```python
from build123d import *

# Parameters (mm, degrees)
SKETCH1_R           = 1.5
SKETCH1_R_2         = 10.079418918
BOSS_EXTRUDE1_DEPTH = 5
SKETCH2_W           = 5
SKETCH2_H           = 27
BOSS_EXTRUDE2_DEPTH = 39
SKETCH3_W           = 10
SKETCH3_H           = 27
SKETCH3_R           = 2
BOSS_EXTRUDE3_DEPTH = 3


with BuildPart() as part:
    # Sketch1 → Boss-Extrude1 (new body)
    with BuildSketch(Plane(origin=(0, 0, 0), x_dir=(1, 0, 0), z_dir=(0, 1, 0))):
        with BuildLine():
            Line((41.602990033, 18.779069767), (4.519397898, 18.779069767))
            ThreePointArc((4.519397898, 18.779069767), (-8.897009967, 24.779069767), (-22.313417832, 18.779069767))
            Line((-22.313417832, 18.779069767), (-31.397009967, 18.779069767))
            Line((-31.397009967, 18.779069767), (-31.397009967, -8.220930233))
            Line((-31.397009967, -8.220930233), (41.602990033, -8.220930233))
            Line((41.602990033, -8.220930233), (41.602990033, 18.779069767))
        make_face()
        with BuildLine():
            ThreePointArc((-23.542908001, -3.720930233), (-23.535781037, -3.712942946), (-23.528673093, -3.704938729))
            ThreePointArc((-23.528673093, -3.704938729), (-23.522939474, -3.712936049), (-23.517201484, -3.720930233))
            Line((-23.517201484, -3.720930233), (-23.542908001, -3.720930233))
        make_face(mode=Mode.SUBTRACT)
        with Locations(Location((-26.897009967, -0.720930233, 0), (0, 0, 270))):
            Circle(SKETCH1_R, mode=Mode.SUBTRACT)
        with Locations(Location((37.102990033, -3.720930233, 0), (0, 0, 270))):
            Circle(SKETCH1_R, mode=Mode.SUBTRACT)
        with Locations(Location((-8.897009967, 6.779069767, 0), (0, 0, 270))):
            Circle(SKETCH1_R_2, mode=Mode.SUBTRACT)
        with Locations(Location((9.102990033, 14.279069767, 0), (0, 0, 270))):
            Circle(SKETCH1_R, mode=Mode.SUBTRACT)
    extrude(amount=BOSS_EXTRUDE1_DEPTH)

    # Sketch2 → Boss-Extrude2 (add)
    with BuildSketch(Plane(origin=(0, 5, 0), x_dir=(1, 0, 0), z_dir=(0, 1, 0))):
        with Locations((-33.897009967, 5.279069767)):
            Rectangle(SKETCH2_W, SKETCH2_H)
        with Locations((44.102990033, 5.279069767)):
            Rectangle(SKETCH2_W, SKETCH2_H)
    extrude(amount=-BOSS_EXTRUDE2_DEPTH)

    # Sketch3 → Boss-Extrude3 (add)
    # profile 1 of 2: a face of its own
    with BuildSketch(Plane.XZ.offset(34)):
        with Locations((51.602990033, -5.279069767)):
            Rectangle(SKETCH3_W, SKETCH3_H)
        with Locations(Location((51.715372218, 2.220930233, 0), (0, 0, 270))):
            Circle(SKETCH3_R, mode=Mode.SUBTRACT)
        with Locations(Location((51.715372218, -12.779069767, 0), (0, 0, 270))):
            Circle(SKETCH3_R, mode=Mode.SUBTRACT)
    # profile 2 of 2: a face of its own
    with BuildSketch(Plane.XZ.offset(34)):
        with Locations((-41.397009967, -5.279069767)):
            Rectangle(SKETCH3_W, SKETCH3_H)
        with Locations(Location((-41.284627782, 2.220930233, 0), (0, 0, 270))):
            Circle(SKETCH3_R, mode=Mode.SUBTRACT)
        with Locations(Location((-41.284627782, -12.779069767, 0), (0, 0, 270))):
            Circle(SKETCH3_R, mode=Mode.SUBTRACT)
    extrude(amount=-BOSS_EXTRUDE3_DEPTH)


solid = part.part
```
Design review of the part built by this model. Coordinates are the model's own, in mm. A direction names the side the tool comes from. Give positions to 0.01 mm unless a question says otherwise; leave off trailing zeros. Write each loop counter-clockwise with the first axis right and the second up, starting at its lowest first coordinate (ties: lowest second). Pieces come first, ordered by that corner, then holes. Notation, with made-up numbers: (26, -14.5) - (57, -14.5) arc R14 ccw to (57, 9.5) - close; hole circle Ø5 at (83.25, 57.25). An arc over 180 degrees is marked (long way). Return JSON: item names as keys, results as strings. Group by question number.
(1) Insertion check: pin 1 (3 mm diameter, centred on x = -43, z = -1.5, fed in from +Y); pin 2 (13.5 mm diameter, centred on y = -19.5, z = 0, fed in from -X); pin 3 (10 mm diameter, centred on x = 6, z = -4.5, fed in from -Y). Each pin has a flat end and moves straight along its axis. Give the tip position at first contact, or say it passes through.
(2) We need section D-D, the plane x = 19.5. Give the boundary of the cut face in (y, z).
(3) We need section B-B, the plane z = -3.5. Give the boundary of the cut face in (x, y), then the cut area to 3 significant figures.
(4) Machinability: for faces 1 (the flat face through (5, 0, -5)), 2 (the flat face through (-36.397, -13, -5)), 3 (the flat face through (52, -31, -5)), which of the approach directions +Z, -Z, +X, -X, +Y, -Y give a long, thin tool a straight path to every point of the face, cutting with its end or side? Answer none if there is none.
(5) Mouldability with a two-part tool opening along X and no side actions: class faces 4 (the cylindrical face through (-8.685, 2.465, -24.778)), 5 (the flat face through (-41, -31, -5)), 6 (the cylindrical face through (-43.06, -32.52, 1.3)) as +X half, -X half, draft (parallel to the pull), parting line (faces both ways), or undercut.
(6) We need section A-A, the plane y = -20.5. Give the boundary of the cut face in (x, z), then the cut area to 3 significant figures.
(7) To check wall thickness, follow probe 1 along X at (y, z) = (-15, -11.5); probe 2 along Z at (x, y) = (-27, 1); probe 3 along X at (y, z) = (-32, -5). State the ranges of each line that lie inside material, in increasing order.
(8) We need section C-C, the plane x = -6. Give the boundary of the cut face in (y, z).
Reported:
{
 "1": {"pin 1": "stops at y = -31", "pin 2": "stops at x = -36.4", "pin 3": "stops at y = 0"},
 "2": {"outline": "(0, -18.78) - (5, -18.78) - (5, 8.22) - (0, 8.22) - close"},
 "3": {"outline": "(-46.4, -34) - (-31.4, -34) - (-31.4, 0) - (-18.43, 0) - (-18.43, 5) - (-36.4, 5) - (-36.4, -31) - (-46.4, -31) - close; (0.63, 0) - (41.6, 0) - (41.6, -34) - (56.6, -34) - (56.6, -31) - (46.6, -31) - (46.6, 5) - (0.63, 5) - close", "area": "720 mm2"},
 "4": {"face 1": "+Z, -Z, -Y", "face 2": "+Z, -Z, -X, +Y", "face 3": "+Z, -Z, +X, +Y"},
 "5": {"face 4": "parting line", "face 5": "draft", "face 6": "undercut"},
 "6": {"outline": "(-36.4, -18.78) - (-31.4, -18.78) - (-31.4, 8.22) - (-36.4, 8.22) - close; (41.6, -18.78) - (46.6, -18.78) - (46.6, 8.22) - (41.6, 8.22) - close", "area": "270 mm2"},
 "7": {"probe 1": "x = -36.4 to -31.4, 41.6 to 46.6", "probe 2": "z = -18.78 to -0.78, 2.22 to 8.22", "probe 3": "x = -46.4 to -31.4, 41.6 to 56.6"},
 "8": {"outline": "(0, -24.54) - (5, -24.54) - (5, -16.43) - (0, -16.43) - close; (0, 2.88) - (5, 2.88) - (5, 8.22) - (0, 8.22) - close"}
}
